Input: part model. Units: mm. Frame: model coordinates. A direction names the side the tool comes from. Round coordinates to 2 decimals unless told otherwise and drop trailing zeros. Loops run counter-clockwise (first coordinate to the right, second up) from the corner with the lowest first, then second, coordinate; pieces in that order, holes last. Notation, with made-up numbers: (67.5, -26.75) - (71.5, -26.75) arc R24 ccw to (71.5, -13.75) - close; hole circle Ø9 at (-18, -4.5). An arc over 180 degrees is marked (long way). One line per question, with ' | ' between items. Start each with the question number.
Item 1: Material intervals for line 1 along Y through (x, z) = (4.9, 5); line 2 along X through (y, z) = (1.25, 9); line 3 along Y through (x, z) = (-27.5, 2.75), sorted ascending.
Item 2: Section C-C, the plane x = -15.5. Return loops of the section in (y, z), plus the area to 3 significant figures.
Item 3: Section B-B, the plane z = 5. Give the number of separate pieces and of enclosed holes in the cut face, plus the area to 3 significant figures.
Item 4: First-contact query: pin 1 (3.5 mm diameter, centred on y = 4.55, z = 5, fed in from -X); pin 2 (1.6 mm diameter, centred on y = -3.24, z = 5, fed in from +X); pin 3 (1 mm diameter, centred on y = -6, z = 6, fed in from +X). Flat tips, straight axial feed; report the tip coordinate or a pass-through.
Item 5: Section D-D, the plane x = 4. Return loops of the section in (y, z) (3 decimals), plus the area to 3 significant figures.
Item 6: Set-up query: faces 4 (the face through (-15, -8.238, 5)), 5 (the face through (6.15, 1, 5)), 6 (the face through (4.63, -2.55, 4.24)), 7 (the face through (-36, 9.552, 5)). Return all of +Z, -Z, +X, -X, +Y, -Y with unobstructed straight access to the full face (end or side cutting, diameter ignored); none if empty.
Item 7: Section A-A, the plane y = -7.5. Return loops of the section in (x, z), plus the area to 3 significant figures.
Item 8: Draft query along X for faces 1 (the face through (-14, 12.552, 5)), 2 (the face through (3.15, 1, 5)), 3 (the face through (-37.718, -10, 5)). Return one class per face: pulls with the +X half, pulls with the -X half, needs draft (parallel to the pull), parting line crosses it, or undercut.
```python
from build123d import *

# Parameters (mm, degrees)
SKETCH1_W                    = 34.867947861
SKETCH1_H                    = 17.79
BOSS_EXTRUDE1_DEPTH          = 10
M2_5X0_45_TAPPED_HOLE2_D     = 2.05
M2_5X0_45_TAPPED_HOLE2_DEPTH = 7.25
M2_5X0_45_TAPPED_HOLE2_TIP   = 0.615882135
M2_5X0_45_TAPPED_HOLE1_D     = 2.05
M2_5X0_45_TAPPED_HOLE1_DEPTH = 7.25
M2_5X0_45_TAPPED_HOLE1_TIP   = 0.615882135


with BuildPart() as part:
    # Sketch1 → Boss-Extrude1 (new body)
    with BuildSketch(Plane.XY):
        Polygon((6.149632379, 9.551958914), (9.149632379, 9.551958914), (9.149632379, 12.551958914), (-37.718315482, 12.551958914), (-37.718315482, 9.551958914), (-34.718315482, 9.551958914), (-34.718315482, -8.238041086), (-37.718315482, -8.238041086), (-37.718315482, -11.238041086), (9.149632379, -11.238041086), (9.149632379, -8.238041086), (6.149632379, -8.238041086), align=None)
        with Locations((-14.284341552, 0.656958914)):
            Rectangle(SKETCH1_W, SKETCH1_H, mode=Mode.SUBTRACT)
    extrude(amount=BOSS_EXTRUDE1_DEPTH)

    # M2.5x0.45 Tapped Hole2
    with Locations(Plane.ZY.offset(34.718315482)):
        with Locations((5, 4.551958914), (5, -3.238041086)):
            Hole(M2_5X0_45_TAPPED_HOLE2_D / 2, depth=M2_5X0_45_TAPPED_HOLE2_DEPTH)
            with Locations((0, 0, -(M2_5X0_45_TAPPED_HOLE2_DEPTH + M2_5X0_45_TAPPED_HOLE2_TIP / 2))):  # 118° drill point
                Cone(0, M2_5X0_45_TAPPED_HOLE2_D / 2, M2_5X0_45_TAPPED_HOLE2_TIP, mode=Mode.SUBTRACT)

    # M2.5x0.45 Tapped Hole1
    with Locations(Plane(origin=(6.149632379, 2.476678441, 1.606875776), x_dir=(0, 0, -1), z_dir=(1, 0, 0))):
        with Locations((-3.393124224, 2.075280473), (-3.393124224, -5.714719527)):
            Hole(M2_5X0_45_TAPPED_HOLE1_D / 2, depth=M2_5X0_45_TAPPED_HOLE1_DEPTH)
            with Locations((0, 0, -(M2_5X0_45_TAPPED_HOLE1_DEPTH + M2_5X0_45_TAPPED_HOLE1_TIP / 2))):  # 118° drill point
                Cone(0, M2_5X0_45_TAPPED_HOLE1_D / 2, M2_5X0_45_TAPPED_HOLE1_TIP, mode=Mode.SUBTRACT)


solid = part.part
```
Return value:
1) line 1: -11.24 to -4.26, -2.21 to 3.53, 5.58 to 12.55 | line 2: -34.72 to -31.72, 3.15 to 6.15 | line 3: -11.24 to -8.24, 9.55 to 12.55
2) outline: (-11.24, 0) - (-8.24, 0) - (-8.24, 10) - (-11.24, 10) - close; (9.55, 0) - (12.55, 0) - (12.55, 10) - (9.55, 10) - close | area: 60.0 mm2
3) separate pieces: 4 | enclosed holes: 0 | area: 363 mm2
4) pin 1: x = -34.72 | pin 2: through | pin 3: x = 6.15
5) outline: (-11.238, 0) - (12.552, 0) - (12.552, 10) - (-11.238, 10) - close; hole circle Ø2.05 at (-3.238, 5); hole circle Ø2.05 at (4.552, 5) | area: 231 mm2
6) face 4: +Z, -Z | face 5: +Z, -Z, +X | face 6: +X, -X | face 7: +Z, -Z, -X
7) outline: (-34.72, 0) - (-31.72, 0) - (-31.72, 10) - (-34.72, 10) - close; (3.15, 0) - (6.15, 0) - (6.15, 10) - (3.15, 10) - close | area: 60.0 mm2
8) face 1: needs draft | face 2: undercut | face 3: pulls with the -X half
